from build123d import *


with BuildPart() as part:
    # Sketch3 → Revolve3 (revolve)
    with BuildSketch(Plane.XY, mode=Mode.PRIVATE) as revolve3_sk:
        with BuildLine():
            Line((-206, -98), (-190, -98))
            Line((-190, -98), (-190, -104))
            Line((-190, -104), (-197, -104))
            ThreePointArc((-197, -104), (-205.900774526, -105.350807815), (-214, -109.281585811))
            Line((-214, -109.281585811), (-221.085945401, -114.154919145))
            ThreePointArc((-221.085945401, -114.154919145), (-231.635573734, -116.203059338), (-240.912230418, -121.628294541))
            Line((-240.912230418, -121.628294541), (-247.316956158, -127))
            Line((-247.316956158, -127), (-265.007764466, -127))
            Line((-265.007764466, -127), (-385.522110558, -146.907802754))
            ThreePointArc((-385.522110558, -146.907802754), (-392.425145491, -147.745592099), (-399.374599409, -147.988228651))
            Line((-399.374599409, -147.988228651), (-439.374599409, -147.988228651))
            Line((-439.374599409, -147.988228651), (-438.509351825, -145.325270406))
            add(Edge.make_bspline(
                [(-438.509351825, -145.325270406), (-438.092908159, -144.043588589), (-435.74371961, -142.389326154), (-433.583616452, -141.988422425), (-432.826378566, -141.988422425)],
                knots=[0, 0, 0, 0, 0.670786836, 1, 1, 1, 1], degree=3))
            Line((-432.826378566, -141.988422425), (-399.326378566, -141.988422425))
            ThreePointArc((-399.326378566, -141.988422425), (-392.891699012, -141.763758951), (-386.5, -140.988028076))
            Line((-386.5, -140.988028076), (-265.5, -121))
            Line((-265.5, -121), (-249.5, -121))
            Line((-249.5, -121), (-234, -108))
            Line((-234, -108), (-218, -108))
            Line((-218, -108), (-206, -98))
        make_face()
    revolve(revolve3_sk.sketch.rotate(Axis((0, 0, 0), (1, 0, 0)), 270), axis=Axis((0, 0, 0), (1, 0, 0)))


solid = part.part
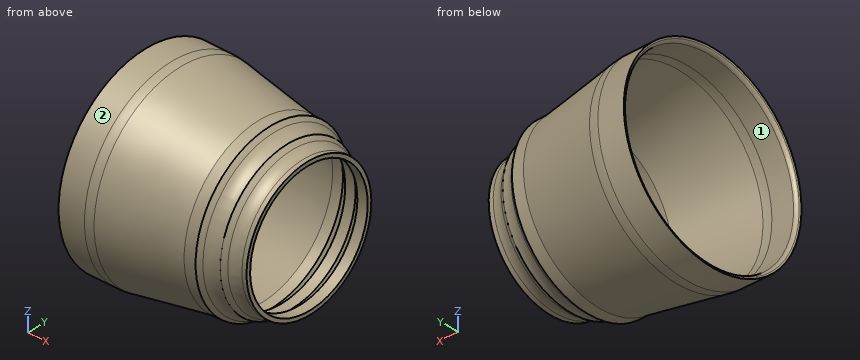
Can you work these out from the model? Positions are in its coordinate system, mm. Face numbers are marked on the shaded views. Coordinates: 2 decimals unless noted, no trailing zeros. Write each loop counter-clockwise with the first axis right and the second up, starting at its lowest first coordinate (ties: lowest second). Pieces come first, ordered by that corner, then holes. Notation, with made-up numbers: (-14, 26) -> (-4, 26) arc R20 ccw to (-4, 40) -> close; hole circle Ø10 at (38, 45.5). An arc over 180 degrees is marked (long way). Write each question's results on one line, items separated by ' | '. Start each with the question number.
Q1. If I drill on probe 1 along Y at (x, z) = (-423, 0); probe 2 along Y at (x, z) = (-259, 0); probe 3 along Z at (x, y) = (-238, -88.5), over which ranges is the centre line in solid material (lowest first)?
Q2. Imagine slicing it at A-A (x = -411.5). Write out the boundary of the cut face in (y, z), then the cut area to 3 significant figures.
Q3. Imagine slicing it at B-B (x = -301). Write out the boundary of the cut face in (y, z).
Q4. We'd pull the mould along Z, two halves only. Please class the marked faces 1 and 2: +Z half, -Z half, draft (parallel to the pull), parting line (faces both ways), or undercut.
Q5. I'm going to push flat-ended pins straight in: pin 1 (10 mm diameter, centred on x = -323.5, y = 68.5, fed in from -Z); pin 2 (12 mm diameter, centred on x = -350, z = -110, fed in from +Y); pin 3 (1 mm diameter, centred on y = 23.5, z = -107.5, fed in from +X). Where does each tip first touch, or does it pass through?
Taken from the geometry:
1) probe 1: y = -147.99 to -141.99, 141.99 to 147.99 | probe 2: y = -127 to -121, 121 to 127 | probe 3: z = -80.23 to -67.58, 67.58 to 80.23
2) outline: circle Ø295.98 at (0, 0); hole circle Ø283.98 at (0, 0) | area: 5,470 mm^2
3) outline: circle Ø265.89 at (0, 0); hole circle Ø253.73 at (0, 0)
4) face 1: undercut | face 2: parting line
5) pin 1: stops at z = -121.17 | pin 2: stops at y = 95.43 | pin 3: stops at x = -214.37
